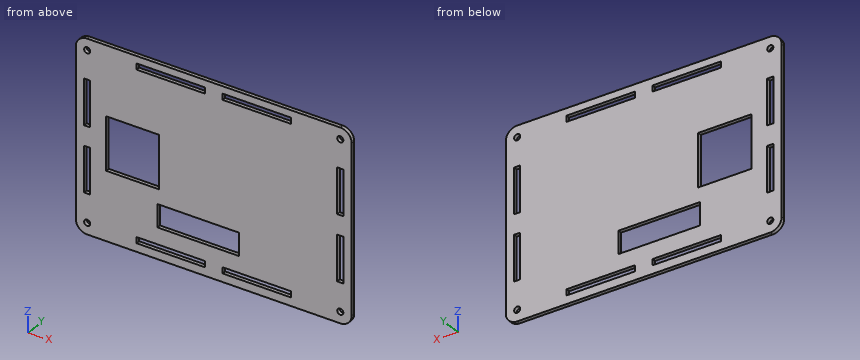
from build123d import *

# Parameters (mm, degrees)
SKETCH1_W           = 145.34
SKETCH1_H           = 100.51
SKETCH1_R           = 1.6
SKETCH1_W_2         = 36
SKETCH1_H_2         = 3.2
SKETCH1_W_3         = 3.2
SKETCH1_H_3         = 24
SKETCH1_W_4         = 28
SKETCH1_H_4         = 28
SKETCH1_W_5         = 43
SKETCH1_H_5         = 12
BOSS_EXTRUDE1_DEPTH = 2
FILLET1_R           = 6
FILLET2_R           = 6
FILLET3_R           = 6


with BuildPart() as part:
    # Sketch1 → Boss-Extrude1 (new body)
    with BuildSketch(Plane(origin=(0, 0, 0), x_dir=(1, 0, 0), z_dir=(0, 1, 0))):
        with Locations((72.67, 50.255)):
            Rectangle(SKETCH1_W, SKETCH1_H)
        with Locations(Location((6, 94.51, 0), (0, 0, 270))):
            Circle(SKETCH1_R, mode=Mode.SUBTRACT)
        with Locations(Location((139.34, 94.51, 0), (0, 0, 270))):
            Circle(SKETCH1_R, mode=Mode.SUBTRACT)
        with Locations(Location((139.34, 6, 0), (0, 0, 270))):
            Circle(SKETCH1_R, mode=Mode.SUBTRACT)
        with Locations(Location((6, 6, 0), (0, 0, 270))):
            Circle(SKETCH1_R, mode=Mode.SUBTRACT)
        with Locations((50, 5.414130674)):
            Rectangle(SKETCH1_W_2, SKETCH1_H_2, mode=Mode.SUBTRACT)
        with Locations((50, 94.51)):
            Rectangle(SKETCH1_W_2, SKETCH1_H_2, mode=Mode.SUBTRACT)
        with Locations((95.34, 94.51)):
            Rectangle(SKETCH1_W_2, SKETCH1_H_2, mode=Mode.SUBTRACT)
        with Locations((95.34, 5.414130674)):
            Rectangle(SKETCH1_W_2, SKETCH1_H_2, mode=Mode.SUBTRACT)
        with Locations((6, 67.51)):
            Rectangle(SKETCH1_W_3, SKETCH1_H_3, mode=Mode.SUBTRACT)
        with Locations((6, 33)):
            Rectangle(SKETCH1_W_3, SKETCH1_H_3, mode=Mode.SUBTRACT)
        with Locations((139.34, 67.51)):
            Rectangle(SKETCH1_W_3, SKETCH1_H_3, mode=Mode.SUBTRACT)
        with Locations((139.34, 33)):
            Rectangle(SKETCH1_W_3, SKETCH1_H_3, mode=Mode.SUBTRACT)
        with Locations((29.946, 50.413)):
            Rectangle(SKETCH1_W_4, SKETCH1_H_4, mode=Mode.SUBTRACT)
        with Locations((64.452, 78.224)):
            Rectangle(SKETCH1_W_5, SKETCH1_H_5, mode=Mode.SUBTRACT)
    extrude(amount=BOSS_EXTRUDE1_DEPTH)

    # Fillet1
    fillet1_edges = [part.edges().sort_by_distance(p)[0] for p in [
        (0, 1, -100.51),
    ]]
    fillet(fillet1_edges, radius=FILLET1_R)

    # Fillet2
    fillet2_edges = [part.edges().sort_by_distance(p)[0] for p in [
        (0, 1, 0),
    ]]
    fillet(fillet2_edges, radius=FILLET2_R)

    # Fillet3
    fillet3_edges = [part.edges().sort_by_distance(p)[0] for p in [
        (145.34, 1, -100.51),
        (145.34, 1, 0),
    ]]
    fillet(fillet3_edges, radius=FILLET3_R)


solid = part.part
Model file for the job. Use its own axes, mm. Coordinates: 2 decimals unless noted, no trailing zeros. Write each loop counter-clockwise with the first axis right and the second up, starting at its lowest first coordinate (ties: lowest second). Pieces come first, ordered by that corner, then holes. Notation, with made-up numbers: (88.5, 65.5) - (95.5, 65.5) arc R21 ccw to (95.5, 91.5) - close; hole circle Ø6 at (-18, -24.5). An arc over 180 degrees is marked (long way). Write each question's results on one line, items separated by ' | '. Start each with the question number.
1) Probe line 1 along X through (y, z) = (1.65, -94.51); line 2 along X through (y, z) = (0.55, -34); line 3 along X through (y, z) = (1.9, -72.5). List the from-to ranges inside material, lowest first. Write a range as from..to.
2) Flat gauge pins, fed straight in: P1, Ø3, axis at x = 6, z = -94.51, coming from the +Y side; P2, Ø5, axis at x = 139.34, z = -94.51, coming from the +Y side; P3, Ø0.6, axis at y = 0.5, z = -4.5, coming from the +X side. Where does each tip first touch, or does it go through?
3) Cut at A-A (x = 73.5). Write the cut outline in (y, z), then the cut area to 3 significant figures.
4) Cut at B-B (z = -23). Write the cut outline in (x, y), then the cut area to 3 significant figures.
5) Cut at C-C (x = 50). Write the cut outline in (y, z), then the cut area to 3 significant figures.
6) Cut at D-D (y = 0.5). Count the separate pieces of the cut face and the enclosed holes in it, then the cut area to 3 significant figures.
Returned:
1) line 1: 0..4.4, 7.6..32, 68..77.34, 113.34..137.74, 140.94..145.34 | line 2: 0..4.4, 7.6..137.74, 140.94..145.34 | line 3: 0..4.4, 7.6..42.95, 85.95..137.74, 140.94..145.34
2) P1: through | P2: y = 2 | P3: x = 145.22
3) outline: (0, -100.51) - (2, -100.51) - (2, -84.22) - (0, -84.22) - close; (0, -72.22) - (2, -72.22) - (2, 0) - (0, 0) - close | area: 177 mm^2
4) outline: (0, 0) - (4.4, 0) - (4.4, 2) - (0, 2) - close; (7.6, 0) - (137.74, 0) - (137.74, 2) - (7.6, 2) - close; (140.94, 0) - (145.34, 0) - (145.34, 2) - (140.94, 2) - close | area: 278 mm^2
5) outline: (0, -100.51) - (2, -100.51) - (2, -96.11) - (0, -96.11) - close; (0, -92.91) - (2, -92.91) - (2, -84.22) - (0, -84.22) - close; (0, -72.22) - (2, -72.22) - (2, -7.01) - (0, -7.01) - close; (0, -3.81) - (2, -3.81) - (2, 0) - (0, 0) - close | area: 164 mm^2
6) separate pieces: 1 | enclosed holes: 14 | area: 12,500 mm^2
